Input: part model. Units: mm. Frame: model coordinates. Give positions to 0.01 mm unless a question says otherwise; leave off trailing zeros. Loops run counter-clockwise (first coordinate to the right, second up) from the corner with the lowest first, then second, coordinate; pieces in that order, holes last. Notation, with made-up numbers: M -3,54 L 42,54 A26 ccw 42,85 Z; hole C 36,11.25 d2. An arc over 180 degrees is marked long. One line per item, written item: value. Start each with the question number.
(1) Ray query, line 1 along X through (y, z) = (-11, -155) (3 decimals); line 2 along Z through (x, y) = (281.5, 372.5); line 3 along Y through (x, z) = (-356.5, 167). Return the intervals inside material, ascending. Write a range as from..to.
(2) Pin query (flat end, axial travel): P1, Ø5, axis at y = -26.5, z = -210, coming from the -X side; P2, Ø4, axis at x = -278, z = -206, coming from the +Y side; P3, Ø16, axis at y = -7, z = 57.5, coming from the -X side. Return the tip coordinate at first contact, or that it passes through.
(3) Section A-A on x = -218. Output: boundary loops of the cut face in (y, z), plus the area to 3 significant figures.
(4) Section B-B on z = 163. Output: boundary loops of the cut face in (x, y) (1 decimal), plus the area to 3 significant figures.
(5) Section D-D on x = -524.5. Output: boundary loops of the cut face in (y, z), plus the area to 3 significant figures.
(6) Section C-C on y = 100. Output: boundary loops of the cut face in (x, z), plus the area to 3 significant figures.
```python
from build123d import *

# Parameters (mm, degrees)
SKETCH6_W                       = 500
SKETCH6_H                       = 431.8
SKETCH6_W_2                     = 460
SKETCH6_H_2                     = 391.8
SKETCH6_W_3                     = 95.25
SKETCH6_W_4                     = 250
SKETCH6_H_3                     = 20
BOSS_EXTRUDE2_DEPTH             = 20
BOSS_EXTRUDE6_START             = -195.9
SKETCH8_R                       = 5
BOSS_EXTRUDE6_DEPTH             = 20
BOSS_EXTRUDE7_START             = 215.9
SKETCH8_6_R                     = 5
BOSS_EXTRUDE7_DEPTH             = 20
BOSS_EXTRUDE8_REACH             = 783.357
SKETCH8_7_R                     = 5
BOSS_EXTRUDE8_DIRECTION_2_REACH = 783.357
BOSS_EXTRUDE9_START             = -195.9
BOSS_EXTRUDE9_DEPTH             = 20
BOSS_EXTRUDE10_START            = 195.9
BOSS_EXTRUDE10_DEPTH            = 20
BOSS_EXTRUDE11_START            = 179.1
SKETCH8_8_R                     = 5
BOSS_EXTRUDE11_DEPTH            = 195.9
BOSS_EXTRUDE12_START            = -375
SKETCH8_9_R                     = 5
BOSS_EXTRUDE12_DEPTH            = 195.9
BOSS_EXTRUDE13_START            = -195.9
BOSS_EXTRUDE13_DEPTH            = 391.8
BOSS_EXTRUDE14_START            = -195.9
BOSS_EXTRUDE14_DEPTH            = 391.8
BOSS_EXTRUDE15_START            = -195.9
SKETCH9_6_R                     = 10
BOSS_EXTRUDE15_DEPTH            = 391.8
BOSS_EXTRUDE16_REACH            = 982.051
SKETCH10_R                      = 10


# Read off the part's stored shape, not the designer's step: Boss-Extrude10, Boss-Extrude14
with BuildPart() as part:
    # Sketch6 → Boss-Extrude2 (new body)
    # profile 1 of 3: a face of its own
    with BuildSketch(Plane(origin=(0, 0, 0), x_dir=(1, 0, 0), z_dir=(0, 1, 0))):
        with Locations((-250, 0)):
            Rectangle(SKETCH6_W, SKETCH6_H)
        with Locations((-250, 0)):
            Rectangle(SKETCH6_W_2, SKETCH6_H_2, mode=Mode.SUBTRACT)
    # profile 2 of 3: a face of its own
    with BuildSketch(Plane(origin=(0, 0, 0), x_dir=(1, 0, 0), z_dir=(0, 1, 0))):
        with Locations((-360, 0)):
            Rectangle(SKETCH6_W_3, SKETCH6_H_2)
    # profile 3 of 3: a face of its own
    with BuildSketch(Plane(origin=(0, 0, 0), x_dir=(1, 0, 0), z_dir=(0, 1, 0))):
        with Locations((-625, 0)):
            Rectangle(SKETCH6_W_4, SKETCH6_H_3)
    extrude(amount=-BOSS_EXTRUDE2_DEPTH)

    # Sketch8 → Boss-Extrude6 (add)
    # profile 1 of 2: a face of its own
    with BuildSketch(Plane.XY.offset(BOSS_EXTRUDE6_START)):
        with BuildLine():
            Line((-2.5, -30), (-2.5, -20))
            Line((-2.5, -20), (-17.5, -20))
            Line((-17.5, -20), (-17.5, -30))
            ThreePointArc((-17.5, -30), (-10, -37.5), (-2.5, -30))
        make_face()
        with Locations((-10, -30)):
            Circle(SKETCH8_R, mode=Mode.SUBTRACT)
    # profile 2 of 2: a face of its own
    with BuildSketch(Plane.XY.offset(BOSS_EXTRUDE6_START)):
        with Locations((-10, -30)):
            Circle(SKETCH8_R)
    extrude(amount=-BOSS_EXTRUDE6_DEPTH)

    # Sketch8<6> → Boss-Extrude7 (add)
    # profile 1 of 2: a face of its own
    with BuildSketch(Plane.XY.offset(BOSS_EXTRUDE7_START)):
        with BuildLine():
            Line((-2.5, -30), (-2.5, -20))
            Line((-2.5, -20), (-17.5, -20))
            Line((-17.5, -20), (-17.5, -30))
            ThreePointArc((-17.5, -30), (-10, -37.5), (-2.5, -30))
        make_face()
        with Locations((-10, -30)):
            Circle(SKETCH8_6_R, mode=Mode.SUBTRACT)
    # profile 2 of 2: a face of its own
    with BuildSketch(Plane.XY.offset(BOSS_EXTRUDE7_START)):
        with Locations((-10, -30)):
            Circle(SKETCH8_6_R)
    extrude(amount=-BOSS_EXTRUDE7_DEPTH)

    # Boss-Extrude8: up to this face of the body (flat: up to its plane)
    boss_extrude8_end = Plane(part.part.faces().sort_by_distance((-166.1875, -10, 195.9))[0])
    # Sketch8<7> → Boss-Extrude8 (add, up to the picked face)
    with BuildSketch(Plane.XY, mode=Mode.PRIVATE) as boss_extrude8_sk1:
        with Locations((-10, -30)):
            Circle(SKETCH8_7_R)
    boss_extrude8_tool1 = split(extrude(boss_extrude8_sk1.sketch, amount=BOSS_EXTRUDE8_REACH, mode=Mode.PRIVATE), bisect_by=boss_extrude8_end, keep=Keep.BOTH, mode=Mode.PRIVATE)
    add(boss_extrude8_tool1.solids().sort_by(Axis((-10, -30, 0), (0, 0, 1)))[0])

    # Boss-Extrude8 direction 2: up to this face of the body (flat: up to its plane)
    boss_extrude8_direction_2_end = Plane(part.part.faces().sort_by_distance((-443.8125, -10, -195.9))[0])
    # Sketch8<7> → Boss-Extrude8 direction 2 (add, up to the picked face)
    with BuildSketch(Plane.XY, mode=Mode.PRIVATE) as boss_extrude8_direction_2_sk1:
        with Locations((-10, -30)):
            Circle(SKETCH8_7_R)
    boss_extrude8_direction_2_tool1 = split(extrude(boss_extrude8_direction_2_sk1.sketch, amount=-BOSS_EXTRUDE8_DIRECTION_2_REACH, mode=Mode.PRIVATE), bisect_by=boss_extrude8_direction_2_end, keep=Keep.BOTH, mode=Mode.PRIVATE)
    add(boss_extrude8_direction_2_tool1.solids().sort_by(Axis((-10, -30, 0), (0, 0, -1)))[0])

    # Sketch9 → Boss-Extrude9 (add)
    with BuildSketch(Plane.XY.offset(BOSS_EXTRUDE9_START)):
        with BuildLine():
            Line((298.618579246, 426.471528727), (0, 0))
            Line((0, 0), (0, -20))
            Line((0, -20), (10.411341011, -20))
            Line((10.411341011, -20), (315.001620132, 415))
            Line((315.001620132, 415), (427.584922624, 480))
            Line((427.584922624, 480), (467.584922624, 410.717967697))
            Line((467.584922624, 410.717967697), (484.9054307, 420.717967697))
            Line((484.9054307, 420.717967697), (434.9054307, 507.320508076))
            Line((434.9054307, 507.320508076), (305.001620132, 432.320508076))
            ThreePointArc((305.001620132, 432.320508076), (301.161755938, 430.103561449), (298.618579246, 426.471528727))
        make_face()
    extrude(amount=-BOSS_EXTRUDE9_DEPTH)

    # Boss-Extrude10 outline → Boss-Extrude10 (add)
    with BuildSketch(Plane.XY.offset(BOSS_EXTRUDE10_START)):
        with BuildLine():
            Line((434.9054307, 507.320508076), (305.001620132, 432.320508076))
            ThreePointArc((305.001620132, 432.320508076), (301.161755938, 430.103561449), (298.618579246, 426.471528727))
            Line((298.618579246, 426.471528727), (0, 0))
            Line((0, 0), (0, -20))
            Line((0, -20), (10.411341011, -20))
            Line((10.411341011, -20), (315.001620132, 415))
            Line((315.001620132, 415), (427.584922624, 480))
            Line((427.584922624, 480), (467.584922624, 410.717967697))
            Line((467.584922624, 410.717967697), (484.9054307, 420.717967697))
            Line((484.9054307, 420.717967697), (434.9054307, 507.320508076))
        make_face()
    extrude(amount=BOSS_EXTRUDE10_DEPTH)

    # Sketch8<8> → Boss-Extrude11 (add)
    with BuildSketch(Plane.XY.offset(BOSS_EXTRUDE11_START)):
        with Locations((-10, -30)):
            Circle(SKETCH8_8_R)
    extrude(amount=BOSS_EXTRUDE11_DEPTH)

    # Sketch8<9> → Boss-Extrude12 (add)
    with BuildSketch(Plane.XY.offset(BOSS_EXTRUDE12_START)):
        with Locations((-10, -30)):
            Circle(SKETCH8_9_R)
    extrude(amount=BOSS_EXTRUDE12_DEPTH)

    # Boss-Extrude14 outline → Boss-Extrude14 (add)
    with BuildSketch(Plane.XY.offset(BOSS_EXTRUDE14_START)):
        with BuildLine():
            ThreePointArc((301.161755938, 430.103561449), (313.203085607, 413.681259926), (305.001620132, 432.320508076))
            Line((305.001620132, 432.320508076), (301.161755938, 430.103561449))
        make_face()
    extrude(amount=BOSS_EXTRUDE14_DEPTH)

    # Sketch9<6> → Boss-Extrude15 (add)
    with BuildSketch(Plane.XY.offset(BOSS_EXTRUDE15_START)):
        with Locations(Location((431.245176662, 493.660254038, 0), (0, 0, 120))):
            Circle(SKETCH9_6_R)
    extrude(amount=BOSS_EXTRUDE15_DEPTH)


with BuildPart() as body_2:
    # Sketch9<4> → Boss-Extrude13 (new body)
    with BuildSketch(Plane.XY.offset(BOSS_EXTRUDE13_START)):
        with BuildLine():
            Line((301.161755938, 430.103561449), (298.618579246, 426.471528727))
            ThreePointArc((298.618579246, 426.471528727), (302.206662098, 414.161374144), (315.001620132, 415))
            ThreePointArc((315.001620132, 415), (317.457036008, 418.426528886), (318.324483178, 422.551780725))
            ThreePointArc((318.324483178, 422.551780725), (314.138351629, 430.8120276), (305.001620132, 432.320508076))
            Line((305.001620132, 432.320508076), (301.161755938, 430.103561449))
        make_face()
    extrude(amount=BOSS_EXTRUDE13_DEPTH)


    add(part.part)  # Boss-Extrude16 merges part
    # Boss-Extrude16: up to this plane
    boss_extrude16_end = Plane(origin=(-17.660444431, 6.427876097, 0), z_dir=(0.939692620785907, -0.3420201433256725, 0))
    # Sketch10 → Boss-Extrude16 (add, up to the surface)
    with BuildSketch(Plane(origin=(0, 0, 0), x_dir=(0, 0, 1), z_dir=(-0.8191520442889914, 0.5735764363510468, 0)), mode=Mode.PRIVATE) as boss_extrude16_sk1:
        with Locations(Location((-205.9, 510.6256051, 0), (0, 0, 90))):
            Circle(SKETCH10_R)
    boss_extrude16_tool1 = split(extrude(boss_extrude16_sk1.sketch, amount=BOSS_EXTRUDE16_REACH, mode=Mode.PRIVATE), bisect_by=boss_extrude16_end, keep=Keep.BOTH, mode=Mode.PRIVATE)
    boss_extrude16 = boss_extrude16_tool1.solids().sort_by_distance((292.882815, 418.280008, -205.9))[0]
    add(boss_extrude16)

    # Mirror1: Boss-Extrude16 across plane
    add(boss_extrude16.mirror(Plane.XY))


solid = body_2.part
```
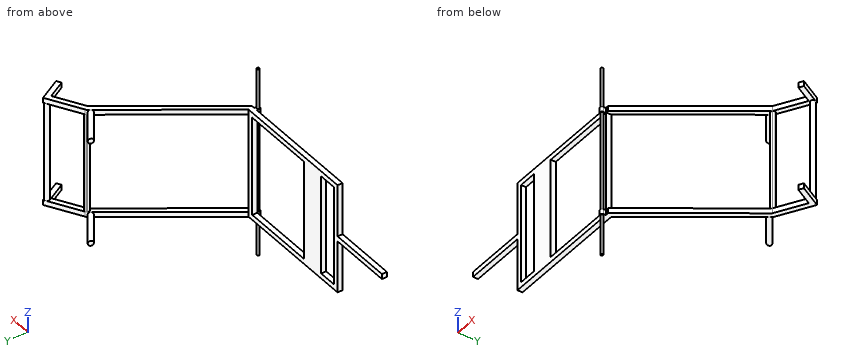
Output values:
1. line 1: x = -500..-480, -407.625..-312.375, -20..0
1. line 2: z = -215.9..-195.9, 195.9..215.9
1. line 3: y = -20..0
2. P1: stops at x = -17.5
2. P2: stops at y = 0
2. P3: stops at x = -500
3. outline: M -20,-215.9 L 0,-215.9 L 0,-195.9 L -20,-195.9 Z; M -20,195.9 L 0,195.9 L 0,215.9 L -20,215.9 Z
3. area: 800 mm²
4. outline: M -500,-20 L -480,-20 L -480,0 L -500,0 Z; M -407.6,-20 L -312.4,-20 L -312.4,0 L -407.6,0 Z; M -20,-20 L 0,-20 L 0,0 L -20,0 Z; C -10,-30 d10; M 301.2,430.1 A10.2 ccw long 305,432.3 Z; C 431.2,493.7 d20
4. area: 3,430 mm²
5. outline: M -20,-10 L 0,-10 L 0,10 L -20,10 Z
5. area: 400 mm²
6. outline: M 70.02,-215.9 L 94.44,-215.9 L 94.44,-195.9 L 70.02,-195.9 Z; M 70.02,195.9 L 94.44,195.9 L 94.44,215.9 L 70.02,215.9 Z
6. area: 977 mm²
